Part model, mm, in its own coordinate system. A direction names the side the tool comes from. Give positions to 0.01 mm unless a question says otherwise; leave off trailing zeros. Order: outer loops, then holes, each group sorted by start corner. A loop starts at its lowest first (then second) coordinate and runs counter-clockwise, first axis right, second up.
1. Mould opens along X. For faces 1 (the flat face through (98.925, -23, 54)), 2 (the flat face through (79.875, -23, 54)), 3 (the flat face through (89, -38.1, 56)), 4 (the flat face through (89.53, -18.78, 107.97)) say: +X half, -X half, draft (parallel to the pull), parting line (faces both ways), or undercut.
2. Which spindle directions (+Z, -Z, +X, -X, +Y, -Y) get a long thin tool onto all of the face, cutting with end or side? Do faces 5 (the flat face through (-110.625, -19, 82)), 6 (the flat face through (-120, 0, 85)), 7 (the flat face through (-120, -38.1, 85)). Say none if no direction does.
3. Slice it at B-B on y = 12. List the corners of the cut face in (x, z), and give its area (3 significant figures).
4. Slice it at C-C on x = -50. List the corners of the cut face in (y, z).
5. Slice it at A-A on z = 11.5. List the corners of the cut face in (x, y).
6. Drop flat-ended pins along their axis: pin 1 Ø5.5 at (x, z) = (-115.5, 115.5) entering from -Y; pin 2 Ø21 at (x, z) = (86, 49.5) entering from +Y; pin 3 Ø10 at (x, y) = (-193.5, -42) entering from +Z. Give the stop position or say it passes through.
7. Probe line 1 (X direction, y = -14, z = 95); line 2 (Z direction, x = -7.5, y = -51); line 3 (Z direction, x = 86, y = -19.05) (3 decimals). List the from-to ranges inside material, lowest first.
from build123d import *

# Parameters (mm, degrees)
F1_DEPTH   = 38.1
F2_R       = 3.175
F1_FACE1_W = 38.1
F1_FACE1_H = 163.5125
F3_DEPTH   = 19.05
F4_R       = 3.175
F5_DEPTH   = 19.05
F7_DEPTH   = 25.4
F9_DEPTH   = 88.9


with BuildPart() as f1:
    # F0 (on Front) → F1 (new body)
    with BuildSketch(Plane.XZ):
        Polygon((79.8746063113, 106.3625), (79.8746063113, 0), (98.9246063113, 0), (98.9246063113, 109.5375), align=None)
        Polygon((98.9246063113, 0), (79.8746063113, 0), (-110.6253936887, 0), (-129.6753936887, 0), (-256.6753936887, 0), (-256.6753936887, -12.7), (124.3246063113, -12.7), (124.3246063113, 0), align=None)
        Polygon((-129.6753936887, 0), (-110.6253936887, 0), (-110.6253936887, 166.6875), (-129.6753936887, 163.5125), align=None)
    extrude(amount=F1_DEPTH)

    # F2 (on face) + F1_face1 (on face) → F3 (cut)
    with BuildSketch(Plane.YZ.offset(98.9246063113)):
        with Locations((-19.05, 50.8)):
            Circle(F2_R)
    with BuildSketch(Plane(origin=(-129.6753936887, -19.05, 81.75625), x_dir=(0, -1, 0), z_dir=(-1, 0, 0))):
        Rectangle(F1_FACE1_W, F1_FACE1_H)
    extrude(amount=-F3_DEPTH, dir=(1, 0, 0), mode=Mode.SUBTRACT)

    # F4 (on face) → F5 (cut)
    with BuildSketch(Plane(origin=(-129.6753936887, 0, 0), x_dir=(0, -1, 0), z_dir=(-1, 0, 0))):
        with Locations((19.05, 50.8)):
            Circle(F4_R)
    extrude(amount=-F5_DEPTH, mode=Mode.SUBTRACT)

    # F6 (on face) → F7 (join)
    with BuildSketch(Plane.XZ.offset(38.1)):
        Polygon((-129.6753936887, 0), (-256.6753936887, 0), (-256.6753936887, -12.7), (124.3246063113, -12.7), (124.3246063113, 0), (98.9246063113, 0), (79.8746063113, 0), (-110.6253936887, 0), align=None)
    extrude(amount=F7_DEPTH)

    # F8 (on face) → F9 (join)
    with BuildSketch(Plane(origin=(0, 0, 0), x_dir=(-1, 0, 0), z_dir=(0, 1, 0))):
        Polygon((-98.9246063113, 0), (-124.3246063113, 0), (-124.3246063113, -12.7), (256.6753936887, -12.7), (256.6753936887, 0), (129.6753936887, 0), (110.6253936887, 0), (-79.8746063113, 0), align=None)
    extrude(amount=F9_DEPTH)


solid = f1.part
Data:
1. face 1: +X half
1. face 2: undercut
1. face 3: draft
1. face 4: undercut
2. face 5: +Z, +Y, -Y
2. face 6: +Z, +X, -X, +Y
2. face 7: +Z, +X, -X, -Y
3. outline: (-256.68, -12.7) - (124.32, -12.7) - (124.32, 0) - (-256.68, 0) - close
3. area: 4,840 mm2
4. outline: (-63.5, -12.7) - (88.9, -12.7) - (88.9, 0) - (-63.5, 0) - close
5. outline: (-129.68, -38.1) - (-110.63, -38.1) - (-110.63, 0) - (-129.68, 0) - close; (79.87, -38.1) - (98.92, -38.1) - (98.92, 0) - (79.87, 0) - close
6. pin 1: stops at y = -38.1
6. pin 2: stops at y = 0
6. pin 3: stops at z = 0
7. line 1: x = -129.68 to -110.63, 79.87 to 98.92
7. line 2: z = -12.7 to 0
7. line 3: z = -12.7 to 47.625, 53.975 to 107.383
